from build123d import *

# Parameters (mm, degrees)
SKETCH1_R           = 5
BOSS_EXTRUDE1_DEPTH = 0.35
SKETCH2_R           = 4.25
SKETCH2_R_2         = 3.75
BOSS_EXTRUDE6_DEPTH = 4.5
SKETCH5_R           = 5
SKETCH5_R_2         = 3.75
BOSS_EXTRUDE7_DEPTH = 0.35
SKETCH9_R           = 2.3
CUT_EXTRUDE5_DEPTH  = 11.4
CUT_EXTRUDE6_DEPTH  = 11.4
CUT_EXTRUDE8_START  = -4.85
CUT_EXTRUDE8_DEPTH  = 4.85
SKETCH12_R          = 0.5
CUT_EXTRUDE9_DEPTH  = 4.85


with BuildPart() as part:
    # Sketch1 → Boss-Extrude1 (new body)
    with BuildSketch(Plane(origin=(0, 0, 0), x_dir=(1, 0, 0), z_dir=(0, 1, 0))):
        with Locations(Location((-49.622774045, -6.018603783, 0), (0, 0, 270))):
            Circle(SKETCH1_R)
    extrude(amount=BOSS_EXTRUDE1_DEPTH)

    # Sketch2 → Boss-Extrude6 (add)
    with BuildSketch(Plane(origin=(0, 0.35, 0), x_dir=(1, 0, 0), z_dir=(0, 1, 0))):
        with Locations(Location((-49.622774045, -6.018603783, 0), (0, 0, 270))):
            Circle(SKETCH2_R)
        with Locations(Location((-49.622774045, -6.018603783, 0), (0, 0, 270))):
            Circle(SKETCH2_R_2, mode=Mode.SUBTRACT)
    extrude(amount=BOSS_EXTRUDE6_DEPTH)

    # Sketch5 → Boss-Extrude7 (add)
    with BuildSketch(Plane(origin=(0, 4.85, 0), x_dir=(1, 0, 0), z_dir=(0, 1, 0))):
        with Locations(Location((-49.622774045, -6.018603783, 0), (0, 0, 270))):
            Circle(SKETCH5_R)
        with Locations(Location((-49.622774045, -6.018603783, 0), (0, 0, 270))):
            Circle(SKETCH5_R_2, mode=Mode.SUBTRACT)
    extrude(amount=BOSS_EXTRUDE7_DEPTH)

    # Sketch9 → Cut-Extrude5 (cut)
    with BuildSketch(Plane(origin=(0, 0.35, 0), x_dir=(1, 0, 0), z_dir=(0, 1, 0))):
        with Locations(Location((-49.622774045, -6.018603783, 0), (0, 0, 270))):
            Circle(SKETCH9_R)
    extrude(amount=-CUT_EXTRUDE5_DEPTH, mode=Mode.SUBTRACT)

    # Sketch10 → Cut-Extrude6 (cut)
    with BuildSketch(Plane.XY):
        Polygon((-43.20579759, 3.8), (-43.20579759, 1.4), (-46.977708805, 1.4), (-46.977708805, 2.6), (-46.977708805, 3.8), align=None)
    extrude(amount=CUT_EXTRUDE6_DEPTH, mode=Mode.SUBTRACT)

    # Sketch11 → Cut-Extrude8 (cut)
    with BuildSketch(Plane(origin=(0, 5.2, 0), x_dir=(1, 0, 0), z_dir=(0, 1, 0)).offset(CUT_EXTRUDE8_START)):
        with BuildLine():
            Line((-53.369890601, -6.165632753), (-54.618929453, -6.21464241))
            ThreePointArc((-54.618929453, -6.21464241), (-53.246537308, -9.463649474), (-50.071032009, -10.998469725))
            Line((-50.071032009, -10.998469725), (-50.91884618, -9.53750944))
            ThreePointArc((-50.91884618, -9.53750944), (-52.656060405, -8.223524158), (-53.369890601, -6.165632753))
        make_face()
    extrude(amount=CUT_EXTRUDE8_DEPTH, mode=Mode.SUBTRACT)

    # Sketch12 → Cut-Extrude9 (cut)
    with BuildSketch(Plane.XY):
        with Locations(Location((-49.621140094, 2.6, 0), (0, 0, 180))):
            Circle(SKETCH12_R)
    extrude(amount=CUT_EXTRUDE9_DEPTH, mode=Mode.SUBTRACT)


solid = part.part
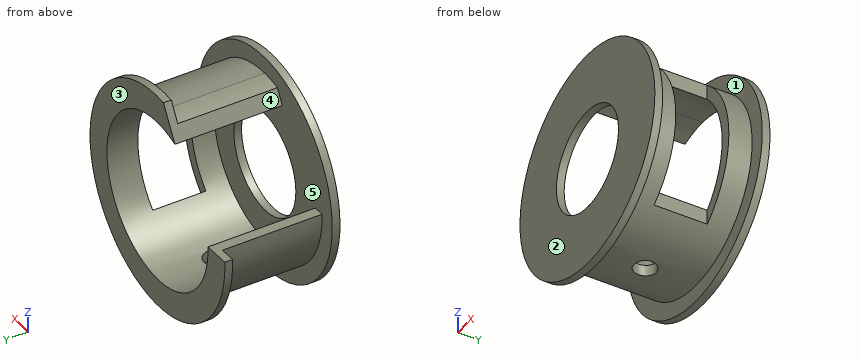
Design review of the part built by this model. Coordinates are the model's own, in mm. Face numbers are marked on the shaded views. A direction names the side the tool comes from. Give positions to 0.01 mm unless a question says otherwise; leave off trailing zeros. Loops run counter-clockwise (first coordinate to the right, second up) from the corner with the lowest first, then second, coordinate; pieces in that order, holes last. Notation, with made-up numbers: M -7.5,51 L 15.5,51 A7 cw 15.5,56 Z; hole C -39.75,-22 d6. An arc over 180 degrees is marked long. Write item = value, one per line.
Q1. Draft analysis for pull direction X (two halves, no side actions). For the marked faces 3, 4 and 5, state which applies: +X half, -X half, draft (parallel to the pull), parting line (faces both ways), or undercut.
Output values:
face_3 = draft
face_4 = -X half
face_5 = undercut
Q2. For the marked faces 1 and 2, list the 3-axis set-ups (+Z, -Z, +X, -X, +Y, -Y) from which the entire face can be reached by the end or side of a thin tool; tool diameter is ignored.
Output values:
face_1 = none
face_2 = +Z, -Z, +X, -X, -Y
Q3. To check wall thickness, follow line 1 (Y direction, x = -49.5, z = 10.5); line 2 (Y direction, x = -45.5, z = 6); line 3 (Y direction, x = -52.5, z = 7). State the ranges of each line that lie inside material, in increasing order. Write a range as [from, to].
Output values:
line_1 = [0, 0.35], [4.85, 5.2]
line_2 = [0, 1.4], [3.8, 5.2]
line_3 = [0, 0.35]
Q4. Insertion check: pin 1 (4 mm diameter, centred on x = -49.62, z = 6.02, fed in from +Y); pin 2 (5 mm diameter, centred on x = -50, z = 5, fed in from +Y); pin 3 (0.7 mm diameter, centred on y = 2, z = 9, fed in from +X); pin 4 (4 mm diameter, centred on x = -48.5, z = 6, fed in from +Y). Each pin has a flat end and moves straight along its axis. Give the tip position at first contact, or say it passes through.
Output values:
pin_1 = through
pin_2 = 0.35
pin_3 = -46.98
pin_4 = 0.35
Q5. We need section A-A (z = 8.5). Give the boundary of the cut face in (x, y).
Output values:
outline = M -53.96,0 L -45.28,0 L -45.28,0.35 L -46.17,0.35 L -46.17,1.4 L -46.81,1.4 L -46.81,0.35 L -53.96,0.35 Z; M -46.81,3.8 L -46.17,3.8 L -46.17,4.85 L -45.28,4.85 L -45.28,5.2 L -46.81,5.2 Z
Q6. We need section B-B (y = 2.6). Give the boundary of the cut face in (x, z), plus the area to 3 significant figures.
Output values:
outline = M -53.87,6.19 A4.25 ccw -50.12,1.8 L -50.12,2.3 A3.75 cw -53.37,6.17 Z; M -50.92,9.54 A3.75 cw -46.98,8.68 L -46.98,9.35 A4.25 ccw -50.55,10.17 Z; M -49.12,1.8 A4.25 ccw -46.98,2.69 L -46.98,3.36 A3.75 cw -49.12,2.3 Z
area = 6.17 mm^2
Q7. We need section D-D (z = 2). Give the boundary of the cut face in (x, y), plus the area to 3 significant figures.
Output values:
outline = M -52.6,0 L -46.65,0 L -46.65,0.35 L -48.24,0.35 L -48.24,4.85 L -46.65,4.85 L -46.65,5.2 L -52.6,5.2 L -52.6,4.85 L -51.01,4.85 L -51.01,0.35 L -52.6,0.35 Z; hole C -49.62,2.6 d1
area = 15.8 mm^2
Q8. We need section C-C (x = -45.75). Give the boundary of the cut face in (y, z).
Output values:
outline = M 0,2.86 L 0.35,2.86 L 0.35,4.27 L 1.4,4.27 L 1.4,7.77 L 0.35,7.77 L 0.35,9.18 L 0,9.18 Z; M 3.8,4.27 L 4.85,4.27 L 4.85,2.86 L 5.2,2.86 L 5.2,9.18 L 4.85,9.18 L 4.85,7.77 L 3.8,7.77 Z
